Here's how the part is built. I have some questions about the finished solid (model axes, mm). Round coordinates to 2 decimals unless told otherwise and drop trailing zeros. Write each loop counter-clockwise with the first axis right and the second up, starting at its lowest first coordinate (ties: lowest second). Pieces come first, ordered by that corner, then holes. Notation, with made-up numbers: (57, 36) - (63, 36) arc R13 cw to (63, 45) - close; hole circle Ø11 at (44, -14.5). An arc over 180 degrees is marked (long way). Return JSON: item names as keys, results as strings. Group by question number.
Autodesk Inventor part; units mm, degrees
ref_plane "YZ Plane" through (0, 0, 0) normal (1, 0, 0) x (0, 1, 0)
ref_plane "XZ Plane" through (0, 0, 0) normal (0, 1, 0) x (-1, 0, 0)
ref_plane "XY Plane" through (0, 0, 0) normal (0, 0, 1) x (1, 0, 0)
sketch "Skizze1" plane through (0, 0, 0) normal (1, 0, 0) x (0, 1, 0)
  line L0 (0, 0) -> (-10, 0) construction
  circle A0 centre (0, 0) radius 1.1
  circle A1 centre (-10, 0) radius 1.1
  arc A2 (-10, 2.5) -> (-10, -2.5) centre (-10, 0) ccw
  line L1 (-10, -2.5) -> (3.4, -2.5)
  line L2 (-10, 2.5) -> (1.4, 2.5)
  arc A3 (3.4, 0.5) -> (1.4, 2.5) centre (1.4, 0.5) ccw
  line L3 (3.4, 0.5) -> (3.4, -2.5)
  dimension "d0" = 10
  dimension "d1" = 2.2
  dimension "d2" = 2.2
  dimension "d3" = 2.5
  dimension "d8" = 2
  dimension "d9" = 3.4
extrude "Extrusion1" add sketch "Skizze1" along normal mid plane 4
chamfer "Fase1" distance 0.5 angle 45 10 edges at (2, 2.8142, 1.9142) (2, -4.3, 2.5) (2, -12.5, 0) (2, -3.3, -2.5) (2, 3.4, -1) (-2, 2.8142, 1.9142) (-2, -4.3, 2.5) (-2, -12.5, 0) (-2, -3.3, -2.5) (-2, 3.4, -1)
sketch "Skizze4" plane through (-1.5, -10, 2.5) normal (0, 0, 1) x (1, 0, 0)
  line L0 (1.5, 16.58) -> (1.5, -5.68) construction
  line L1 (0, 0) -> (3, 0) construction
  line L2 (0.75, 0.4) -> (2.25, 0.4)
  line L3 (2.25, 0.4) -> (2.25, 0)
  line L4 (2.25, 0) -> (0.75, 0)
  line L5 (0.75, 0) -> (0.75, 0.4)
  line L6 (0.75, 0.4) -> (2.25, 0) construction
  line L7 (2.25, 0.4) -> (0.75, 0) construction
  point P0 (1.5, 10)
  point P1 (1.5, 0.2)
  point P2 (1.5, 0)
  dimension "d23" = 0.4
  dimension "d24" = 1.5
extrude "Extrusion3" cut sketch "Skizze4" against normal blind 0.2
pattern_linear "Rechteckige Anordnung1" count 3 spacing 1 along (0, 1, 0) of "Extrusion3"
equation "\"d2\" = d1"
properties part number "Chipanschlag T1.5"
1) If we mould it in two halves opening along Y, with no side actions, what happens to faces 1 (the cylindrical face through (-0.03, 1.05, -0.33)), 2 (the cylindrical face through (-0.028, -8.984, 0.421)), 3 (the flat face through (0, 3.4, -1)), 4 (the flat face through (2, -5, 0))? For each: released by +Y, released by -Y, zero draft, split by the parting line, or undercut.
2) Imagine slicing it at A-A (z = 0). Please give me the cut outline in (x, y).
3) Will these pins go through, and if not, where does the flat tip stop? pin 1 Ø1 at (x, z) = (-1.5, -1.5) entering from -Y; pin 2 Ø2.5 at (y, z) = (0, 0) entering from +X.
4) Imagine slicing it at C-C (y = 0). Please give me the cut outline in (x, z), plus the area to 3 significant figures.
5) Imagine slicing it at D-D (y = -8.25). Please give me the cut outline in (x, z).
6) Imagine slicing it at B-B (x = -1.25). Please give me the cut outline in (y, z), plus the area to 3 significant figures.
7) I need wall thicknesses on line 1 along Z through (x, y) = (-0.15, 0); line 2 along Y through (x, z) = (-1.05, -0.9); line 3 along Y through (x, z) = (0.6, 0.7). Which ranges of each line are inside material? Lowest first, please.
Results found:
{
 "1": {"face 1": "undercut", "face 2": "undercut", "face 3": "released by +Y", "face 4": "zero draft"},
 "2": {"outline": "(-2, -12) - (-1.5, -12.5) - (1.5, -12.5) - (2, -12) - (2, -11.1) - (-2, -11.1) - close; (-2, -8.9) - (2, -8.9) - (2, -1.1) - (-2, -1.1) - close; (-2, 1.1) - (2, 1.1) - (2, 2.9) - (1.5, 3.4) - (-1.5, 3.4) - (-2, 2.9) - close"},
 "3": {"pin 1": "stops at y = -12.29", "pin 2": "stops at x = 2"},
 "4": {"outline": "(-2, -2) - (-1.5, -2.5) - (1.5, -2.5) - (2, -2) - (2, -1.1) - (-2, -1.1) - close; (-2, 1.1) - (2, 1.1) - (2, 2) - (1.5, 2.5) - (-1.5, 2.5) - (-2, 2) - close", "area": "10.7 mm²"},
 "5": {"outline": "(-2, -2) - (-1.5, -2.5) - (1.5, -2.5) - (2, -2) - (2, 2) - (1.5, 2.5) - (-1.5, 2.5) - (-2, 2) - close"},
 "6": {"outline": "(-10, -2.5) - (3.4, -2.5) - (3.4, 0.5) arc R2 ccw to (1.4, 2.5) - (-10, 2.5) arc R2.5 ccw to start; hole circle Ø2.2 at (-10, 0); hole circle Ø2.2 at (0, 0)", "area": "68.4 mm²"},
 "7": {"line 1": "z = -2.5 to -1.1, 1.1 to 2.5", "line 2": "y = -12.33 to -10.63, -9.37 to -0.63, 0.63 to 3.4", "line 3": "y = -12.4 to -10.85, -9.15 to -0.85, 0.85 to 3.39"}
}
